```python
from build123d import *

# Parameters (mm, degrees)
SKETCH_R     = 14.5
PAD_DEPTH    = 53
PAD001_DEPTH = 10
SKETCH001_W  = 16
SKETCH001_H  = 16
POCKET_DEPTH = 70


with BuildPart() as part:
    # Sketch → Pad (new body)
    with BuildSketch(Plane.XY):
        Circle(SKETCH_R)
    extrude(amount=PAD_DEPTH)

    # Sketch002 → Pad001 (join)
    with BuildSketch(Plane.XY.offset(53)):
        Polygon((21, 0), (10.5, 18.186533), (-10.5, 18.186533), (-21, 0), (-10.5, -18.186533), (10.5, -18.186533), align=None)
    extrude(amount=PAD001_DEPTH)

    # Sketch001 → Pocket (cut)
    with BuildSketch(Plane.XY):
        Rectangle(SKETCH001_W, SKETCH001_H)
    extrude(amount=POCKET_DEPTH, mode=Mode.SUBTRACT)


with BuildPart() as part_1:
    # Body placement: moved
    add(part.part.moved(Location((50, 50, -3))))


solid = part_1.part
```
Work out the finished part from the listing and answer in its coordinate system (mm). A direction names the side the tool comes from. Give positions to 0.01 mm unless a question says otherwise; leave off trailing zeros. Loops run counter-clockwise (first coordinate to the right, second up) from the corner with the lowest first, then second, coordinate; pieces in that order, holes last. Notation, with made-up numbers: (-1, 42.25) -> (44, 42.25) arc R12 cw to (44, 61.25) -> close; hole circle Ø1 at (29.25, 87.25). An arc over 180 degrees is marked (long way). Put each result on its own line as item: value. Start each with the question number.
Item 1: The part is cut by section A-A (z = 54). Give the vertices of the cut face in (x, y), then the cut area to 3 significant figures.
Item 2: Each of these flat-tipped pins is pushed along its axis until it touches: P1, Ø8, axis at x = 56.5, z = 27, coming from the +Y side; P2, Ø1, axis at y = 49, z = 14.5, coming from the -X side; P3, Ø2, axis at y = 57, z = 4.5, coming from the -X side. Where does it stop, or does it pass through?
Item 3: The part is cut by section D-D (y = 63). Give the vertices of the cut face in (x, z), then the cut area to 3 significant figures.
Item 4: The part is cut by section B-B (x = 50). Give the vertices of the cut face in (y, z).
Item 5: Which of the six approach directions +Z, -Z, +X, -X, +Y, -Y give full straight-line access (tool end or side, diameter ignored) to faces 1 (the face through (50, 31.813, 55)), 2 (the face through (50, 58, 28)), 3 (the face through (62.3, 58.2, 50))?
Item 6: Find the intervals of material crossed by L1, parallel to Z at x = 48, y = 66; L2, parallel to X at y = 49, z = 19; L3, parallel to X at y = 44, z = 42.5, in increasing order. Write a range as [from, to].
Item 7: The mould has two halves that part along Y. Classify faces 4 (the face through (50, 42, 28)), 5 (the face through (34.18, 41.03, 54.93)), 6 (the face through (59, 50, -3)), 7 (the face through (58, 50, 28)): released by +Y, released by -Y, zero draft, split by the parting line, or undercut.
Item 8: The part is cut by section C-C (z = 37.5). Give the vertices of the cut face in (x, y).
Answers below:
1. outline: (29, 50) -> (39.5, 31.81) -> (60.5, 31.81) -> (71, 50) -> (60.5, 68.19) -> (39.5, 68.19) -> close; hole (42, 42) -> (58, 42) -> (58, 58) -> (42, 58) -> close
1. area: 890 mm2
2. P1: y = 64.28
2. P2: x = 35.51
2. P3: x = 36.8
3. outline: (36.51, 50) -> (43.58, 50) -> (43.58, -3) -> (56.42, -3) -> (56.42, 50) -> (63.49, 50) -> (63.49, 60) -> (36.51, 60) -> close
3. area: 951 mm2
4. outline: (31.81, 50) -> (35.5, 50) -> (35.5, -3) -> (42, -3) -> (42, 60) -> (31.81, 60) -> close; (58, -3) -> (64.5, -3) -> (64.5, 50) -> (68.19, 50) -> (68.19, 60) -> (58, 60) -> close
5. face 1: +Z, -Z, +X, -X, -Y
5. face 2: +Z, -Z
5. face 3: -Z
6. L1: [50, 60]
6. L2: [35.53, 42], [58, 64.47]
6. L3: [36.8, 42], [58, 63.2]
7. face 4: undercut
7. face 5: released by -Y
7. face 6: zero draft
7. face 7: undercut
8. outline: circle Ø29 at (50, 50); hole (42, 42) -> (58, 42) -> (58, 58) -> (42, 58) -> close
